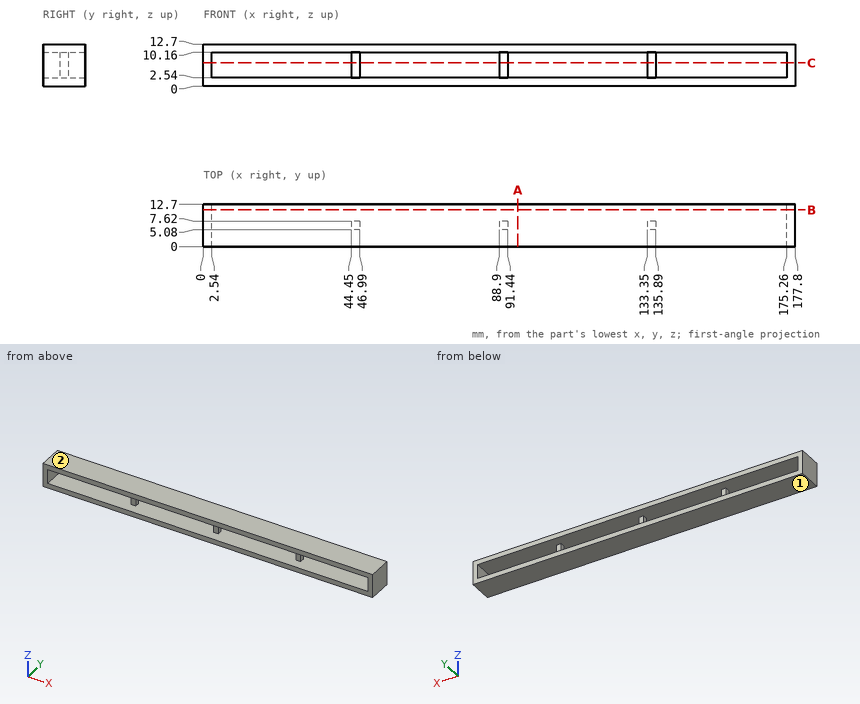
Study the drawing (mm; zero at the part's minimum x, y, z) and answer. Coordinates: 2 decimals unless noted, no trailing zeros. Loops run counter-clockwise (first coordinate to the right, second up) from the corner with the lowest first, then second, coordinate; pieces in that order, holes last. Notation, with made-up numbers: (-29, 12) -> (-19, 12) arc R8 cw to (-19, 25) -> close; hole circle Ø5 at (80, 81). An arc over 180 degrees is marked (long way). Answer in a Markdown table with one row per item. Add a question column.
1. The part is cut by section A-A, the plane x = 94.5. Write down the section's boundary in (y, z).
2. Flat-ended cylindrical pins translate along their axes: P1, Ø2, axis at x = 134.5, z = 6, coming from the +Y side; P2, Ø3, axis at x = 134, z = 5.5, coming from the -Y side. Find the tip coordinate at first contact, or state that the pin passes through.
3. Consider line 1 (Z direction, x = 157, y = 5.75); line 2 (X direction, y = 2, z = 2.75); line 3 (X direction, y = 5.25, z = 5.5). Determine where each line is inside the solid, lowest interval first. Write a range as [from, to].
4. The part is cut by section B-B, the plane y = 11. Write down the section's boundary in (x, z), then the cut area to 3 significant figures.
5. Determine the mould class of the marked faces 1 and 2 for opening direction Z: +Z half, -Z half, draft (parallel to the pull), parting line (faces both ways), or undercut.
6. The part is cut by section C-C, the plane z = 7. Write down the section's boundary in (x, y), then the cut area to 3 significant figures.
Answer below:
| question | item | result |
|---|---|---|
| 1 | outline | (0, 0) -> (12.7, 0) -> (12.7, 2.54) -> (0, 2.54) -> close; (0, 10.16) -> (12.7, 10.16) -> (12.7, 12.7) -> (0, 12.7) -> close |
| 2 | P1 | y = 7.62 |
| 2 | P2 | y = 5.08 |
| 3 | line 1 | [0, 2.54], [10.16, 12.7] |
| 3 | line 2 | [0, 2.54], [175.26, 177.8] |
| 3 | line 3 | [0, 2.54], [44.45, 46.99], [88.9, 91.44], [133.35, 135.89], [175.26, 177.8] |
| 4 | outline | (0, 0) -> (177.8, 0) -> (177.8, 12.7) -> (0, 12.7) -> close; hole (2.54, 2.54) -> (175.26, 2.54) -> (175.26, 10.16) -> (2.54, 10.16) -> close |
| 4 | area | 942 mm2 |
| 5 | face 1 | -Z half |
| 5 | face 2 | +Z half |
| 6 | outline | (0, 0) -> (2.54, 0) -> (2.54, 12.7) -> (0, 12.7) -> close; (44.45, 5.08) -> (46.99, 5.08) -> (46.99, 7.62) -> (44.45, 7.62) -> close; (88.9, 5.08) -> (91.44, 5.08) -> (91.44, 7.62) -> (88.9, 7.62) -> close; (133.35, 5.08) -> (135.89, 5.08) -> (135.89, 7.62) -> (133.35, 7.62) -> close; (175.26, 0) -> (177.8, 0) -> (177.8, 12.7) -> (175.26, 12.7) -> close |
| 6 | area | 83.9 mm2 |
